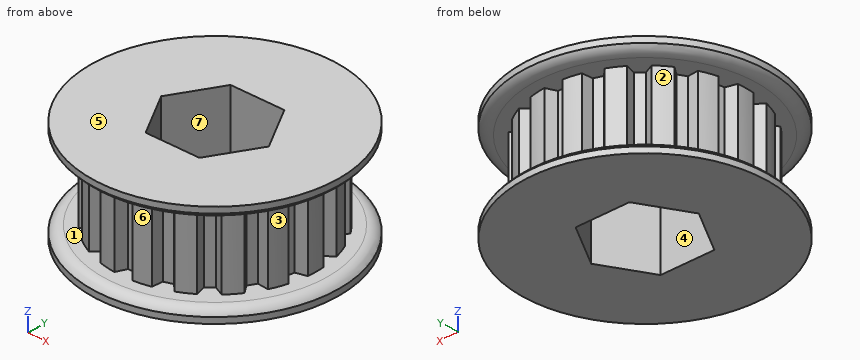
```python
from build123d import *

# Parameters (mm, degrees)
CUT_EXTRUDE1_START = 2.2987
CUT_EXTRUDE1_DEPTH = 10.922
CIRPATTERN1_COUNT  = 18
SKETCH4_R          = 2.0828
CUT_EXTRUDE2_DEPTH = 27.762350537
CUT_EXTRUDE3_DEPTH = 1.5621
CIRPATTERN2_COUNT  = 2
CIRPATTERN2_ANGLE  = 90
CUT_EXTRUDE4_DEPTH = 33.175459463
SKETCH8_R          = 13.842582523
CUT_EXTRUDE5_DEPTH = 29.537230639


with BuildPart() as part:
    # Sketch2 → Revolve1 (revolve)
    with BuildSketch(Plane(origin=(0, 0, 0), x_dir=(0, 0, -1), z_dir=(1, 0, 0)), mode=Mode.PRIVATE) as revolve1_sk:
        with BuildLine():
            Line((-10.3124, 4.7625), (10.3124, 4.7625))
            Line((10.3124, 4.7625), (10.3124, 17.4625))
            Line((10.3124, 17.4625), (9.46785, 17.4625))
            ThreePointArc((9.46785, 17.4625), (8.847668679, 16.777633999), (8.6233, 15.88135))
            Line((8.6233, 15.88135), (8.6233, 14.3002))
            Line((8.6233, 14.3002), (-2.2987, 14.3002))
            Line((-2.2987, 14.3002), (-2.2987, 15.88135))
            ThreePointArc((-2.2987, 15.88135), (-2.523068679, 16.777633999), (-3.14325, 17.4625))
            Line((-3.14325, 17.4625), (-3.9878, 17.4625))
            Line((-3.9878, 17.4625), (-3.9878, 10.3124))
            Line((-3.9878, 10.3124), (-10.3124, 10.3124))
            Line((-10.3124, 10.3124), (-10.3124, 4.7625))
        make_face()
    revolve(revolve1_sk.sketch.rotate(Axis((0, 0, 10.3124), (0, 0, -1)), 90), axis=Axis((0, 0, 10.3124), (0, 0, -1)))

    # Sketch3 → Cut-Extrude1 (cut)
    with BuildSketch(Plane.XY.offset(CUT_EXTRUDE1_START)):
        with BuildLine():
            Line((-0.635, 12.842092967), (0.635, 12.842092967))
            Line((0.635, 12.842092967), (1.287830721, 14.242092967))
            ThreePointArc((1.287830721, 14.242092967), (0, 14.3002), (-1.287830721, 14.242092967))
            Line((-1.287830721, 14.242092967), (-0.635, 12.842092967))
        make_face()
    cut_extrude1 = extrude(amount=-CUT_EXTRUDE1_DEPTH, mode=Mode.SUBTRACT)

    # CirPattern1: Cut-Extrude1 ×18 about axis
    cirpattern1_axis = Axis((0, 0, 0), (0, 0, 1))
    for i in range(1, CIRPATTERN1_COUNT):
        add(cut_extrude1.rotate(cirpattern1_axis, i * 360 / CIRPATTERN1_COUNT), mode=Mode.SUBTRACT)

    # Sketch4 → Cut-Extrude2 (cut, through all)
    with BuildSketch(Plane(origin=(0, 0, 0), x_dir=(1, 0, 0), z_dir=(0, 1, 0))):
        with Locations(Location((0, -7.1501, 0), (0, 0, 90))):
            Circle(SKETCH4_R)
    cut_extrude2 = extrude(amount=CUT_EXTRUDE2_DEPTH, mode=Mode.SUBTRACT)

    # Sketch5 → Revolve2 (revolve)
    with BuildSketch(Plane.XY.offset(7.1501), mode=Mode.PRIVATE) as revolve2_sk:
        Polygon((1.5748, 10.099878114), (2.0828, 9.591878114), (2.0828, 5.3975), (1.4478, 4.7625), (0, 4.7625), (0, 10.099878114), align=None)
    revolve2 = revolve(revolve2_sk.sketch.rotate(Axis((0, 0, 7.1501), (0, 1, 0)), 90), axis=Axis((0, 0, 7.1501), (0, 1, 0)))

    # Sketch6 → Cut-Extrude3 (cut)
    with BuildSketch(Plane(origin=(0, 10.099878114, 0), x_dir=(1, 0, 0), z_dir=(0, 1, 0))):
        Polygon((0, -5.947594859), (-1.0414, -6.54884743), (-1.0414, -7.75135257), (0, -8.352605141), (1.0414, -7.75135257), (1.0414, -6.54884743), align=None)
    cut_extrude3 = extrude(amount=-CUT_EXTRUDE3_DEPTH, mode=Mode.SUBTRACT)

    # CirPattern2: Cut-Extrude2, Revolve2, Cut-Extrude3 ×2 about axis
    cirpattern2_axis = Axis((0, 0, 0), (0, 0, -1))
    add([cut_extrude2.rotate(cirpattern2_axis, i * CIRPATTERN2_ANGLE / (CIRPATTERN2_COUNT - 1)) for i in range(1, CIRPATTERN2_COUNT)], mode=Mode.SUBTRACT)
    add([revolve2.rotate(cirpattern2_axis, i * CIRPATTERN2_ANGLE / (CIRPATTERN2_COUNT - 1)) for i in range(1, CIRPATTERN2_COUNT)])
    add([cut_extrude3.rotate(cirpattern2_axis, i * CIRPATTERN2_ANGLE / (CIRPATTERN2_COUNT - 1)) for i in range(1, CIRPATTERN2_COUNT)], mode=Mode.SUBTRACT)

    # Sketch7 → Cut-Extrude4 (cut, through all)
    with BuildSketch(Plane(origin=(0, 0, -10.3124), x_dir=(-1, 0, 0), z_dir=(0, 0, -1))):
        Polygon((3.812821178, -6.604), (7.625642355, 0), (3.812821178, 6.604), (-3.812821178, 6.604), (-7.625642355, 0), (-3.812821178, -6.604), align=None)
    extrude(amount=-CUT_EXTRUDE4_DEPTH, mode=Mode.SUBTRACT)

    # Sketch8 → Cut-Extrude5 (cut, through all)
    with BuildSketch(Plane.XY.offset(3.9878)):
        Circle(SKETCH8_R)
    extrude(amount=CUT_EXTRUDE5_DEPTH, mode=Mode.SUBTRACT)


solid = part.part
```
Part model, mm, in its own coordinate system. Face numbers are marked on the shaded views. A direction names the side the tool comes from. Give positions to 0.01 mm unless a question says otherwise; leave off trailing zeros. Order: outer loops, then holes, each group sorted by start corner. A loop starts at its lowest first (then second) coordinate and runs counter-clockwise, first axis right, second up. Notation, with made-up numbers: (52.5, 58) - (77.5, 58) arc R15 cw to (77.5, 76) - close; hole circle Ø11 at (-6.75, 75). An arc over 180 degrees is marked (long way). Use one line per item in the form item = value.
Item 1: Which spindle directions (+Z, -Z, +X, -X, +Y, -Y) get a long thin tool onto all of the face, cutting with end or side? Do the marked faces 1, 2 and 3. Say none if no direction does.
Solution:
face_1 = none
face_2 = -X, +Y
face_3 = +X, -Y
Item 2: Two-plate mould, pull along X, no slides. Class the marked faces 4, 5, 6 and 7: released by +X, released by -X, zero draft, split by the parting line, or undercut.
Solution:
face_4 = undercut
face_5 = zero draft
face_6 = released by +X
face_7 = undercut
Item 3: Slice it at A-A on x = 0. Give the cut face in (y, z), and give its area (3 significant figures).
Solution:
outline = (-17.46, -10.31) - (-6.6, -10.31) - (-6.6, 3.99) - (-17.46, 3.99) - (-17.46, 3.14) arc R1.9 ccw to (-15.88, 2.3) - (-12.84, 2.3) - (-12.84, -8.62) - (-15.88, -8.62) arc R1.9 ccw to (-17.46, -9.47) - close; (6.6, -10.31) - (17.46, -10.31) - (17.46, -9.47) arc R1.9 ccw to (15.88, -8.62) - (12.84, -8.62) - (12.84, 2.3) - (15.88, 2.3) arc R1.9 ccw to (17.46, 3.14) - (17.46, 3.99) - (6.6, 3.99) - close
area = 208 mm2
Item 4: Probe probe 1 along Z at (x, y) = (-15, -2); probe 2 along Y at (x, z) = (3.5, 0.75); probe 3 along X at (y, z) = (4.5, -4.75). List the from-to ranges inside material, lowest first. Write a range as from..to.
Solution:
probe_1 = -10.31..-8.62, 2.3..3.99
probe_2 = -13.87..-6.6, 6.6..13.87
probe_3 = -13.57..-5.03, 5.03..13.57
Item 5: Pin check, flat tips, straight feed: pin 1 Ø1 at (x, z) = (0.5, -5.5) entering from +Y; pin 2 Ø8.5 at (x, z) = (1.5, -2) entering from -Y; pin 3 Ø1 at (x, z) = (0, -1) entering from -Y. Stop position of each tip, or through.
Solution:
pin_1 = 13.62
pin_2 = -14.24
pin_3 = -12.84
